```python
from build123d import *

# Parameters (mm, degrees)
SKETCH3_W          = 31.75
SKETCH3_H          = 31.75
SKETCH3_W_2        = 12.7
SKETCH3_H_2        = 15.875
CUT_EXTRUDE1_DEPTH = 8.509


with BuildPart() as part:
    # Sketch1 → Revolve1 (revolve)
    with BuildSketch(Plane.XY):
        Polygon((-9.525, 0), (-9.525, 7.9375), (71.4248, 7.9375), (71.4248, 25.52065), (112.395, 25.52065), (112.395, 0), align=None)
    revolve(axis=Axis((112.395, 0, 0), (-1, 0, 0)))

    # Sketch2 → Revolve2 (revolve)
    with BuildSketch(Plane.XY):
        with BuildLine():
            Line((-31.75, 0), (-31.75, 5.59435))
            Line((-31.75, 5.59435), (-30.99435, 6.35))
            Line((-30.99435, 6.35), (-13.2334, 6.35))
            Line((-13.2334, 6.35), (-12.726366704, 5.842966704))
            ThreePointArc((-12.726366704, 5.842966704), (-12.190743755, 5.485074892), (-11.558933409, 5.3594))
            Line((-11.558933409, 5.3594), (-11.176, 5.3594))
            ThreePointArc((-11.176, 5.3594), (-10.008566704, 5.842966704), (-9.525, 7.0104))
            Line((-9.525, 7.0104), (-9.525, 0))
            Line((-9.525, 0), (-31.75, 0))
        make_face()
    revolve(axis=Axis((-9.525, 0, 0), (-1, 0, 0)))

    # Sketch3 → Cut-Extrude1 (cut)
    with BuildSketch(Plane(origin=(-10.16, 0, 0), x_dir=(0, 0, -1), z_dir=(1, 0, 0))):
        Rectangle(SKETCH3_W, SKETCH3_H)
        Rectangle(SKETCH3_W_2, SKETCH3_H_2, mode=Mode.SUBTRACT)
    extrude(amount=CUT_EXTRUDE1_DEPTH, mode=Mode.SUBTRACT)


solid = part.part
```
Model file for the job. Use its own axes, mm. A direction names the side the tool comes from. Give positions to 0.01 mm unless a question says otherwise; leave off trailing zeros. Write each loop counter-clockwise with the first axis right and the second up, starting at its lowest first coordinate (ties: lowest second). Pieces come first, ordered by that corner, then holes. Notation, with made-up numbers: (80.25, -19.5) - (126.25, -19.5) arc R13 cw to (126.25, 1.5) - close; hole circle Ø2 at (4.5, -13). An arc over 180 degrees is marked (long way). One line per question, with ' | ' between items. Start each with the question number.
(1) Wall check: line 1 along X through (y, z) = (9, 22) (3 decimals); line 2 along X through (y, z) = (5, 4) (3 decimals); line 3 along Y through (x, z) = (92, -12). Give the ranges that are in metal, low to high. Write a range as from..to.
(2) Pin check, flat tips, straight feed: P1, Ø6.5, axis at x = -7.5, y = 2.5, coming from the -Z side; P2, Ø0.5, axis at y = -1.5, z = 7, coming from the -X side; P3, Ø6.5, axis at x = -5.5, y = -2, coming from the +Z side. Stop position of each tip, or through.
(3) Slice it at D-D on x = 52. Write the cut outline in (y, z) (1 decimal), plus the area to 3 significant figures.
(4) 3-axis set-ups, long thin cutter, end or side, ignore diameter. For faces 5 (the face through (-21.99, -1.38, 6.2)), 6 (the face through (-9.525, 7.3, 0.4)), 7 (the face through (-9.525, -7.3, 0)), 8 (the face through (-6, 0, 6.35)), 9 (the face through (-6, 0, -6.35)): which of +Z, -Z, +X, -X, +Y, -Y reach the whole face in a straight line?
(5) Two-plate mould, pull along X, no slides. Class faces 1 (the face through (112.395, 0, 0)), 2 (the face through (71.425, 6, -6)), 3 (the face through (92.197, -5.532, 24.914)), 4 (the face through (-11.365, -5.354, -0.236)): +X half, -X half, draft (parallel to the pull), parting line (faces both ways), or undercut.
Results below:
1) line 1: 71.425..112.395 | line 2: -9.641..112.395 | line 3: -22.52..22.52
2) P1: z = -6.35 | P2: x = -1.65 | P3: z = 6.35
3) outline: circle Ø15.9 at (0, 0) | area: 198 mm^2
4) face 5: -X | face 6: -X, +Y | face 7: -X, -Y | face 8: +Z, -X, +Y, -Y | face 9: -Z, -X, +Y, -Y
5) face 1: +X half | face 2: -X half | face 3: draft | face 4: undercut
